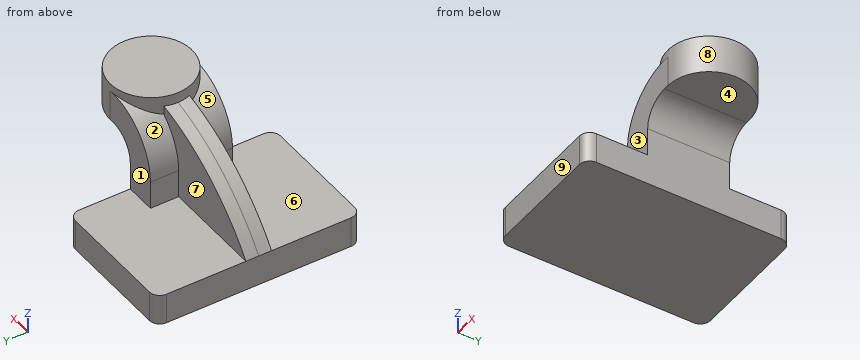
from build123d import *

# Parameters (mm, degrees)
F1_DEPTH = 63.5
F2_DEPTH = 25.4
F3_DEPTH = 7.9375
F5_R     = 6.35


with BuildPart() as f1:
    # F0 (on Front) → F1 (new body, symmetric)
    with BuildSketch(Plane.XZ):
        Polygon((-41.275, -9.525), (41.275, -9.525), (41.275, 9.525), (22.225, 9.525), (-41.275, 9.525), align=None)
    extrude(amount=F1_DEPTH, both=True)

    # F0 (on Front) → F2 (join, symmetric)
    with BuildSketch(Plane.XZ):
        with BuildLine():
            Line((22.225, 9.525), (41.275, 9.525))
            Line((41.275, 9.525), (41.275, 27.0002))
            ThreePointArc((41.275, 27.0002), (45.92468, 38.22552), (57.15, 42.8752))
            Line((57.15, 42.8752), (60.325, 42.8752))
            Line((60.325, 42.8752), (60.325, 61.9252))
            Line((60.325, 61.9252), (57.15, 61.9252))
            ThreePointArc((57.15, 61.9252), (32.454296, 51.695904), (22.225, 27.0002))
            Line((22.225, 27.0002), (22.225, 9.525))
        make_face()
    extrude(amount=F2_DEPTH, both=True)

    # F0 (on Front) → F3 (join, symmetric)
    with BuildSketch(Plane.XZ):
        with BuildLine():
            add(Edge.make_bspline(
                [(-41.275, 9.525), (-19.508036, 40.293224), (20.560727, 63.729674), (57.15, 61.9252)],
                knots=[0, 0, 0, 0, 111.504536, 111.504536, 111.504536, 111.504536], degree=3))
            Line((-41.275, 9.525), (22.225, 9.525))
            Line((22.225, 9.525), (22.225, 27.0002))
            ThreePointArc((22.225, 27.0002), (32.454296, 51.695904), (57.15, 61.9252))
        make_face()
    extrude(amount=F3_DEPTH, both=True)

    # F0 (on Front) → F4 (revolve)
    with BuildSketch(Plane.XZ):
        Polygon((60.325, 66.675), (60.325, 61.9252), (60.325, 42.8752), (85.666397, 42.8752), (85.666397, 66.675), align=None)
    revolve(axis=Axis((60.325, 0, 52.3875), (0, 0, 1)))

    # F5
    f5_edges = [f1.edges().sort_by_distance(p)[0] for p in [
        (-41.275, -63.5, 0),
        (41.275, -63.5, 0),
        (41.275, 63.5, 0),
        (-41.275, 63.5, 0),
    ]]
    fillet(f5_edges, radius=F5_R)


solid = f1.part
Work out the finished part from the listing and answer in its coordinate system (mm). Face numbers are marked on the shaded views. A direction names the side the tool comes from. Give positions to 0.01 mm unless a question says otherwise; leave off trailing zeros. Write each loop counter-clockwise with the first axis right and the second up, starting at its lowest first coordinate (ties: lowest second). Pieces come first, ordered by that corner, then holes. Notation, with made-up numbers: (67, -5) - (118, -5) arc R6 ccw to (118, -1) - close; hole circle Ø3 at (30.25, 69). An arc over 180 degrees is marked (long way). One line per item, written item: value. Start each with the question number.
1. For the marked faces 1, 2, 3, 4 and 5, determine the directions among +Z, -Z, +X, -X, +Y, -Y from which every point of the face is accessible in a straight line to the end or side of a thin tool.
2. Find section B-B (y = -15). Write down the section's boundary in (x, z) (3 decimals), then the cut area to 3 significant figures.
3. Consider probe 1 along X at (y, z) = (26, -4) (3 decimals); probe 2 along Y at (x, z) = (16, 36); probe 3 along Y at (x, z) = (33, 15). Determine where each line is inside the solid, lowest interval first.
4. For a pull along Y with two mould halves and no side action, classify the marked faces 6, 7, 8 and 9 as +Y half, -Y half, draft (parallel to the pull), parting line (faces both ways), or undercut.
5. Find section C-C (x = 77). Write down the section's boundary in (y, z) (3 decimals), then the cut area to 3 significant figures.
6. Find section A-A (z = 0). Write down the section's boundary in (x, y) (3 decimals), then the cut area to 3 significant figures.
7. Find section D-D (y = -32.5). Write down the section's boundary in (x, z) (3 decimals), then the cut area to 3 significant figures.
8. Given pin 1 (6 mm diameter, centred on x = -17.5, y = 32.5, fed in from +Z) (3 decimals); pin 2 (8.5 mm diameter, centred on y = -13, z = 21.5, fed in from -X) (3 decimals); pin 3 (11.5 mm diameter, centred on x = 40.5, z = 43.5, fed in from -Y), each flat-ended and moving along its own axis, determine where each tip first touches the part or whether it passes through.
Geometry results:
1. face 1: +Z, +X, -X, +Y
1. face 2: +Z, -X, +Y
1. face 3: +Z, +X, -X, -Y
1. face 4: -Z, +X, +Y, -Y
1. face 5: +Z, -X, -Y
2. outline: (-41.275, -9.525) - (41.275, -9.525) - (41.275, 27) arc R15.875 cw to (57.15, 42.875) - (80.75, 42.875) - (80.75, 66.675) - (39.9, 66.675) - (39.9, 57.368) arc R34.925 ccw to (22.225, 27) - (22.225, 9.525) - (-41.275, 9.525) - close
2. area: 3,330 mm2
3. probe 1: -41.275 to 41.275
3. probe 2: -7.94 to 7.94
3. probe 3: -25.4 to 25.4
4. face 6: draft
4. face 7: +Y half
4. face 8: parting line
4. face 9: -Y half
5. outline: (-19.082, 42.875) - (19.082, 42.875) - (19.082, 66.675) - (-19.082, 66.675) - close
5. area: 908 mm2
6. outline: (-41.275, -57.15) arc R6.35 ccw to (-34.925, -63.5) - (34.925, -63.5) arc R6.35 ccw to (41.275, -57.15) - (41.275, 57.15) arc R6.35 ccw to (34.925, 63.5) - (-34.925, 63.5) arc R6.35 ccw to (-41.275, 57.15) - close
6. area: 10,400 mm2
7. outline: (-41.275, -9.525) - (41.275, -9.525) - (41.275, 9.525) - (-41.275, 9.525) - close
7. area: 1,570 mm2
8. pin 1: z = 9.525
8. pin 2: x = 22.225
8. pin 3: y = -25.4
